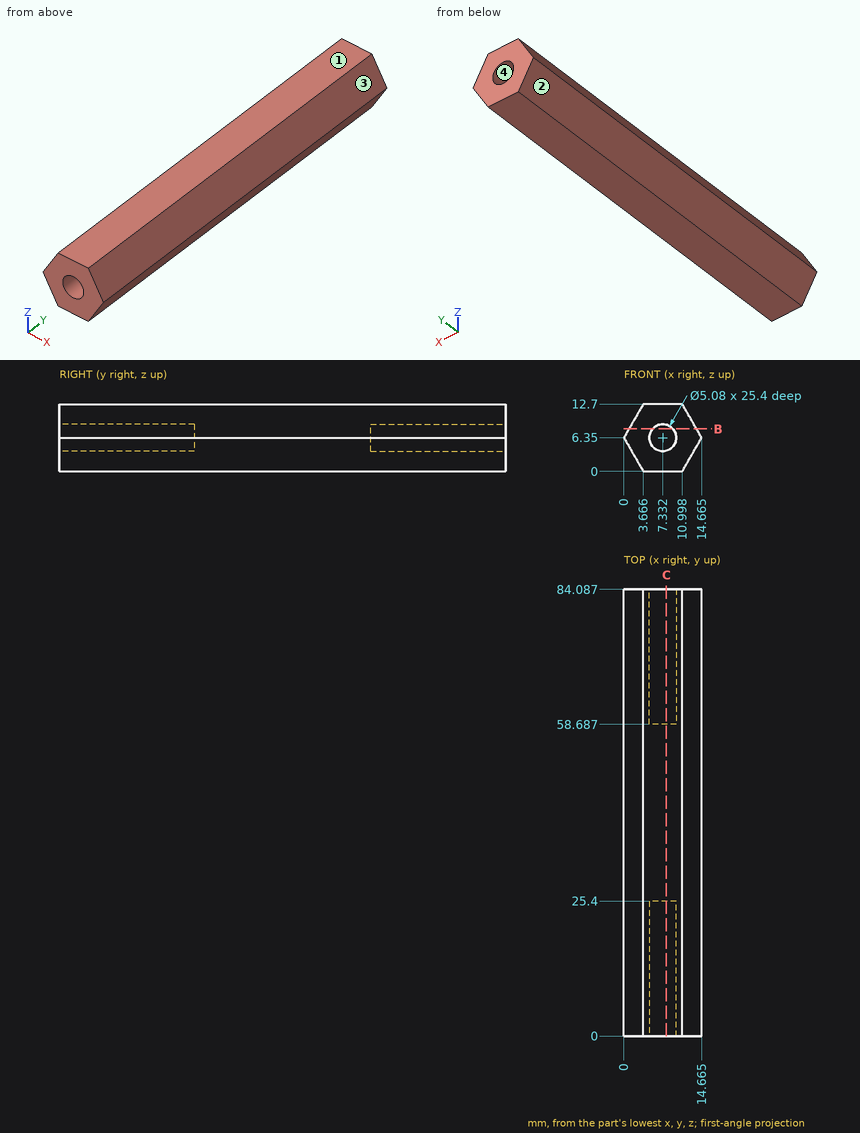
Answer from the drawing. Dimensions are ordinates in mm from the lowest x, y and z of the part. Round coordinates to 2 decimals unless told otherwise and drop trailing zeros. Loops run counter-clockwise (first coordinate to the right, second up) from the corner with the lowest first, then second, coordinate; pieces in that order, holes last.
1) For a pull along X with two mould halves and no side action, classify the marked faces 1, 2, 3 and 4 as released by +X, released by -X, zero draft, split by the parting line, or undercut.
Outcome:
face 1: zero draft
face 2: released by -X
face 3: released by +X
face 4: undercut
2) Given P1, Ø1.5, axis at y = 70, z = 5, coming from the -X side; P2, Ø1.5, axis at y = 38.5, z = 1.5, coming from the -X side; P3, Ø4.5, axis at x = 7.33, z = 6.35, coming from the +Y side, each flat-ended and moving along its own axis, determine where each tip first touches the part or whether it passes through.
Outcome:
P1: stops at x = 0.35
P2: stops at x = 2.37
P3: stops at y = 58.69
3) A cutting plane is placed at B-B on z = 8. Determine the outline of the cut face in (x, y).
Outcome:
outline: (0.95, 0) - (5.4, 0) - (5.4, 25.4) - (9.26, 25.4) - (9.26, 0) - (13.71, 0) - (13.71, 84.09) - (9.26, 84.09) - (9.26, 58.69) - (5.4, 58.69) - (5.4, 84.09) - (0.95, 84.09) - close
4) A cutting plane is placed at C-C on x = 8. Determine the outline of the cut face in (y, z), plus the area to 3 significant figures.
Outcome:
outline: (0, 0) - (84.09, 0) - (84.09, 3.9) - (58.69, 3.9) - (58.69, 8.8) - (84.09, 8.8) - (84.09, 12.7) - (0, 12.7) - (0, 8.8) - (25.4, 8.8) - (25.4, 3.9) - (0, 3.9) - close
area: 819 mm2
5) Consider line 1 (Z direction, x = 6.5, y = 16); line 2 (Y direction, x = 8, z = 7.25); line 3 (X direction, y = 56, z = 2.75) (1 decimal). Determine where each line is inside the solid, lowest interval first.
Outcome:
line 1: z = 0 to 3.95, 8.75 to 12.7
line 2: y = 25.4 to 58.69
line 3: x = 2.1 to 12.6
